Autodesk Inventor part; units mm, degrees
ref_plane "YZ Plane" through (0, 0, 0) normal (1, 0, 0) x (0, 1, 0)
ref_plane "XZ Plane" through (0, 0, 0) normal (0, 1, 0) x (-1, 0, 0)
ref_plane "XY Plane" through (0, 0, 0) normal (0, 0, 1) x (1, 0, 0)
sketch "Boceto1" plane through (0, 0, 0) normal (0, 0, 1) x (1, 0, 0)
  line L0 (8.5, -4) -> (-8.5, -4)
  line L1 (-12.5, -4) -> (-12.5, 4)
  line L2 (-8.5, 4) -> (8.5, 4)
  line L3 (12.5, 4) -> (12.5, -4)
  line L4 (-12.5, 0) -> (-8.5, 0)
  arc A0 (-8.5, 4) -> (-8.5, -4) centre (-8.5, 0) ccw
  line L5 (12.5, 0) -> (8.5, 0)
  arc A1 (8.5, -4) -> (8.5, 4) centre (8.5, 0) ccw
  point P0 (0, 0)
  dimension "d6" = 25
  dimension "d7" = 8
  dimension "d8" = 4
  dimension "d9" = 4
extrude "Extrusión2" add sketch "Boceto1" along normal blind 6
properties part number "Chaveta 25"
Source: CAD feature listing. Evaluate the final solid. Frame: model axes, mm. Give positions to 0.01 mm unless a question says otherwise; leave off trailing zeros. Order: outer loops, then holes, each group sorted by start corner. A loop starts at its lowest first (then second) coordinate and runs counter-clockwise, first axis right, second up. Notation, with made-up numbers: (38.5, 12.25) -> (57.5, 12.25) arc R23 cw to (57.5, 33.25) -> close; hole circle Ø6 at (-23, -9). An arc over 180 degrees is marked (long way). Use a Markdown table: item, result.
Q1. Material intervals for line 1 (X direction, y = 3, z = 5.75); line 2 (X direction, y = 2.75, z = 5.3); line 3 (Y direction, x = -10.75, z = 2.2), sorted ascending. Write a range as [from, to].
A:
| item | result |
|---|---|
| line 1 | [-11.15, 11.15] |
| line 2 | [-11.4, 11.4] |
| line 3 | [-3.31, 3.31] |
Q2. Section B-B (y = -1.75). Return the cut outline in (x, z), and give its area (3 significant figures).
A:
| item | result |
|---|---|
| outline | (-12.1, 0) -> (12.1, 0) -> (12.1, 6) -> (-12.1, 6) -> close |
| area | 145 mm^2 |
Q3. Section A-A (z = 3.3). Return the cut outline in (x, y).
A:
| item | result |
|---|---|
| outline | (-8.5, -4) -> (8.5, -4) arc R4 ccw to (8.5, 4) -> (-8.5, 4) arc R4 ccw to start |
